Geometry check sheet. Reference: the model listing, model coordinates, mm. A direction names the side the tool comes from. Coordinates: 2 decimals unless noted, no trailing zeros. Loops run counter-clockwise (first coordinate to the right, second up) from the corner with the lowest first, then second, coordinate; pieces in that order, holes last.
from build123d import *

# Parameters (mm, degrees)
F1_DEPTH = 12
F3_D     = 2
F3_DEPTH = 7.34
F3_TIP   = 0.600860619


with BuildPart() as f1:
    # F0 (on Front) → F1 (new body)
    with BuildSketch(Plane.XZ):
        with BuildLine():
            Line((-10, 0), (0, 0))
            Line((0, 0), (0, 13))
            Line((0, 13), (-3.4696699141, 9.5303300859))
            Line((-3.4696699141, 9.5303300859), (-4.5303300859, 10.5909902577))
            ThreePointArc((-4.5303300859, 10.5909902577), (-7.3415141503, 12.3415141503), (-5.5909902577, 9.5303300859))
            Line((-5.5909902577, 9.5303300859), (-4.5303300859, 8.4696699141))
            Line((-4.5303300859, 8.4696699141), (-8, 5))
            Line((-8, 5), (-10, 5))
            Line((-10, 5), (-10, 0))
        make_face()
    extrude(amount=F1_DEPTH)

    # F3
    with Locations(Plane(origin=(-10, 0, 0), x_dir=(0, -1, 0), z_dir=(-1, 0, 0))):
        with Locations((6, 2.5)):
            Hole(F3_D / 2, depth=F3_DEPTH)
            with Locations((0, 0, -(F3_DEPTH + F3_TIP / 2))):  # 118° drill point
                Cone(0, F3_D / 2, F3_TIP, mode=Mode.SUBTRACT)


solid = f1.part
(1) Sectioned sample at A-A on x = -9. Record the cut outline in (y, z), and give its area (3 significant figures).
Findings:
outline: (-12, 0) - (0, 0) - (0, 5) - (-12, 5) - close; hole circle Ø2 at (-6, 2.5)
area: 56.9 mm2
(2) Access from +Z, -Z, +X, -X, +Y, -Y to the whole of each face (thin tool, end or side, straight path). Record for faces 1 (the flat face through (-9, -6, 5)), 2 (the flat face through (0, -6, 6)), 3 (the flat face through (-2, -6, 11)), 4 (the flat face through (-6, -6, 7)), 5 (the cylindrical face through (-6.3, -7, 2.5)).
Findings:
face 1: +Z, -X, +Y, -Y
face 2: +Z, -Z, +X, +Y, -Y
face 3: +Z, +Y, -Y
face 4: -X, +Y, -Y
face 5: -X
(3) Gauge pin test, flat ends, axial feed: pin 1 Ø6 at (y, z) = (-4, 11) entering from -X; pin 2 Ø1.6 at (x, y) = (-9.5, -7.5) entering from +Z. Record the tip position at first contact, or that the pin passes through.
Findings:
pin 1: stops at x = -7.84
pin 2: stops at z = 5
(4) Sectioned sample at B-B on z = 12. Record the cut outline in (x, y), and give its area (3 significant figures).
Findings:
outline: (-7.61, -12) - (-4.67, -12) - (-4.67, 0) - (-7.61, 0) - close; (-1, -12) - (0, -12) - (0, 0) - (-1, 0) - close
area: 47.2 mm2
(5) Sectioned sample at D-D on y = -1.5. Record the cut outline in (x, z), and give its area (3 significant figures).
Findings:
outline: (-10, 0) - (0, 0) - (0, 13) - (-3.47, 9.53) - (-4.53, 10.59) arc R1.7 ccw (long way) to (-5.59, 9.53) - (-4.53, 8.47) - (-8, 5) - (-10, 5) - close
area: 93.2 mm2
(6) Scan lines: L1, parallel to Y at x = -8, z = 2.5; L2, parallel to Z at x = -7, y = -6; L3, parallel to Z at x = -5, y = -6. Record each from-to range of solid material in increasing order.
Findings:
L1: y = -12 to -7, -5 to 0
L2: z = 0 to 1.5, 3.5 to 6, 9.67 to 12.61
L3: z = 0 to 1.5, 3.5 to 8, 8.94 to 12.4
(7) Sectioned sample at C-C on x = -6. Record the cut outline in (y, z), and give its area (3 significant figures).
Findings:
outline: (-12, 0) - (0, 0) - (0, 7) - (-12, 7) - close; (-12, 9.45) - (0, 9.45) - (0, 12.83) - (-12, 12.83) - close; hole circle Ø2 at (-6, 2.5)
area: 122 mm2
(8) Draft check along X on faces 6 (the conical face through (-2.16, -5.83, 2.51)), 7 (the flat face through (-4, 0, 5)), 8 (the flat face through (-3.99, -5.92, 10.05)). Enter one of: +X half, -X half, draft (parallel to the pull), parting line (faces both ways), or undercut.
Findings:
face 6: -X half
face 7: draft
face 8: undercut
